CAD build for the part. Positions are in the model's coordinates, mm. A direction names the side the tool comes from. Give positions to 0.01 mm unless a question says otherwise; leave off trailing zeros. Order: outer loops, then holes, each group sorted by start corner. A loop starts at its lowest first (then second) coordinate and runs counter-clockwise, first axis right, second up.
Item 1: Band-saw the part on B-B on x = 0. Give the cut face in (y, z), plus the area to 3 significant figures.
Item 2: Band-saw the part on C-C on y = 22.5. Give the cut face in (x, z), plus the area to 3 significant figures.
Item 3: Band-saw the part on A-A on z = 0. Give the cut face in (x, y).
Item 4: Band-saw the part on D-D on y = 122.5. Give the cut face in (x, z).
Item 5: Flat gauge pins, fed straight in: P1, Ø6, axis at y = 111.5, z = 2.5, coming from the +X side; P2, Ø1, axis at x = 12.5, z = -16, coming from the +Y side; P3, Ø1, axis at x = 0.5, y = 86, coming from the +Z side. Where does each tip first touch, or does it go through?
Item 6: Which spindle directions (+Z, -Z, +X, -X, +Y, -Y) get a long thin tool onto all of the face, cutting with end or side? Do faces 1 (the cylindrical face through (-0.867, 80.193, 3.905)), 2 (the cylindrical face through (23.846, 10.14, -7.509)). Say none if no direction does.
Item 7: Wall check: L1, parallel to Y at x = -10, z = -1; L2, parallel to X at y = 25.5, z = -13; L3, parallel to Y at x = -6, z = 22.5. Give the ranges that are in metal, low to high.
```python
from build123d import *

# Parameters (mm, degrees)
CHAMFER_1_SIZE = 1


with BuildPart() as part:
    # Эскиз1 → Повернуть1 (revolve)
    with BuildSketch(Plane.XY):
        Polygon((0, 0), (25, 0), (25, 20), (15, 30), (4, 30), (4, 130), (0, 130), align=None)
    revolve(axis=Axis((0, 0, 0), (0, 1, 0)))

    # Фаска1
    chamfer_1_edges = [part.edges().sort_by_distance(p)[0] for p in [
        (-4, 130, 0),
    ]]
    chamfer(chamfer_1_edges, length=CHAMFER_1_SIZE)


solid = part.part
```
The answers:
1. outline: (0, -25) - (20, -25) - (30, -15) - (30, -4) - (129, -4) - (130, -3) - (130, 3) - (129, 4) - (30, 4) - (30, 15) - (20, 25) - (0, 25) - close
1. area: 2,200 mm2
2. outline: circle Ø45 at (0, 0)
2. area: 1,590 mm2
3. outline: (-25, 0) - (25, 0) - (25, 20) - (15, 30) - (4, 30) - (4, 129) - (3, 130) - (-3, 130) - (-4, 129) - (-4, 30) - (-15, 30) - (-25, 20) - close
4. outline: circle Ø8 at (0, 0)
5. P1: stops at x = 4
5. P2: stops at y = 25.2
5. P3: stops at z = 4
6. face 1: +Y
6. face 2: +Y, -Y
7. L1: y = 0 to 30
7. L2: x = -14.53 to 14.53
7. L3: y = 0 to 21.71
